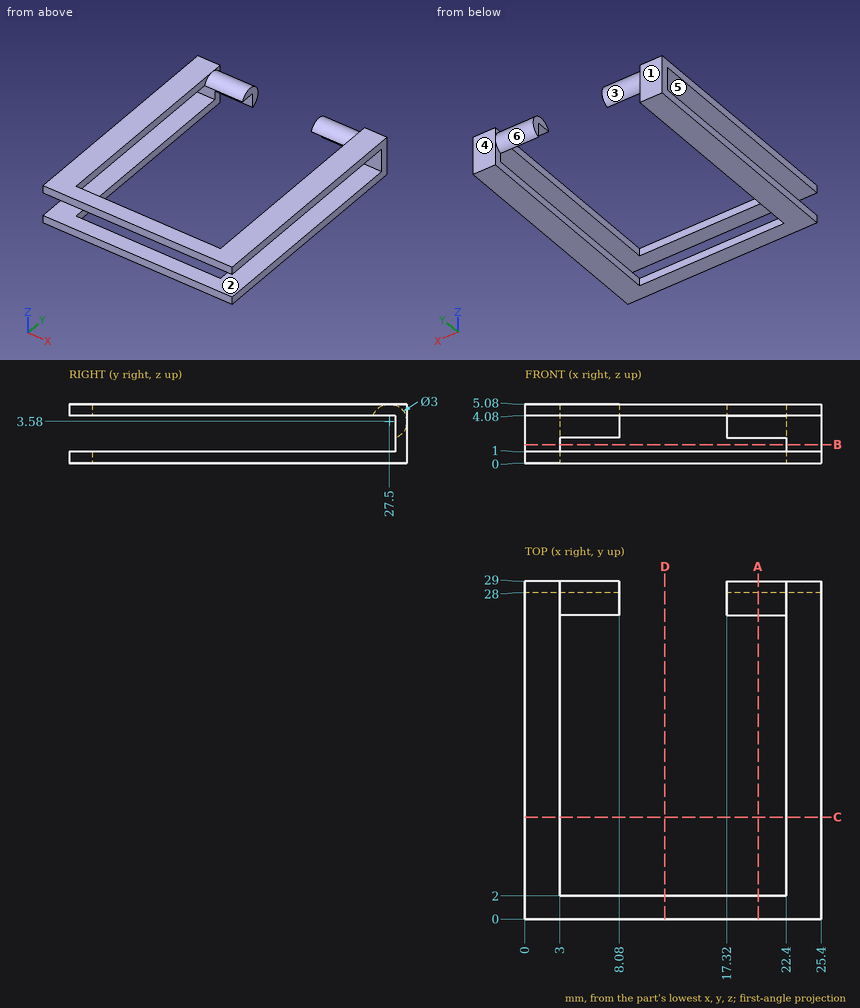
Answer from the drawing. Dimensions are ordinates in mm from the lowest x, y and z of the part. A direction names the side the tool comes from. Give positions to 0.01 mm unless a question says otherwise; leave off trailing zeros. Loops run counter-clockwise (first coordinate to the right, second up) from the corner with the lowest first, then second, coordinate; pieces in that order, holes last. Notation, with made-up numbers: (53, 64) - (59, 64) arc R20 cw to (59, 83) - close; hole circle Ø11 at (89, -31). An arc over 180 degrees is marked (long way). Write each question's results on one line, items separated by ' | '.
1. Find section B-B, the plane z = 1.6. Write down the section's boundary in (x, y), then the cut area to 3 significant figures.
Resolved:
outline: (0, 28) - (3, 28) - (3, 29) - (0, 29) - close; (22.4, 28) - (25.4, 28) - (25.4, 29) - (22.4, 29) - close | area: 6.00 mm^2
2. Which of the six approach directions +Z, -Z, +X, -X, +Y, -Y give full straight-line access (tool end or side, diameter ignored) to the marked faces 4, 5 and 6?
Resolved:
face 4: +Z, -Z, +X, -X, +Y | face 5: +X, -X, -Y | face 6: none
3. For a pull along Y with two mould halves and no side action, classify the marked faces 1, 2 and 3 as +Y half, -Y half, draft (parallel to the pull), parting line (faces both ways), or undercut.
Resolved:
face 1: +Y half | face 2: draft | face 3: undercut
4. Flat-ended cylindrical pins translate along their axes: P1, Ø1.5, axis at x = 22, z = 2, coming from the -Y side; P2, Ø0.5, axis at x = 13.5, z = 0.5, coming from the +Y side; P3, Ø0.9, axis at y = 27.5, z = 4, coming from the -X side. Find the tip coordinate at first contact, or state that the pin passes through.
Resolved:
P1: stops at y = 28 | P2: stops at y = 2 | P3: stops at x = 0
5. Find section C-C, the plane y = 8.75. Write down the section's boundary in (x, z), then the cut area to 3 significant figures.
Resolved:
outline: (0, 0) - (3, 0) - (3, 1) - (0, 1) - close; (0, 4.08) - (3, 4.08) - (3, 5.08) - (0, 5.08) - close; (22.4, 0) - (25.4, 0) - (25.4, 1) - (22.4, 1) - close; (22.4, 4.08) - (25.4, 4.08) - (25.4, 5.08) - (22.4, 5.08) - close | area: 12.0 mm^2
6. Consider probe 1 along Z at (x, y) = (2, 18.75); probe 2 along X at (y, z) = (23.5, 4.25); probe 3 along Y at (x, z) = (15, 4.55). Determine where each line is inside the solid, lowest interval first. Write a range as from..to.
Resolved:
probe 1: z = 0..1, 4.08..5.08 | probe 2: x = 0..3, 22.4..25.4 | probe 3: y = 0..2
7. Find section D-D, the plane x = 12. Write down the section's boundary in (y, z).
Resolved:
outline: (0, 0) - (2, 0) - (2, 1) - (0, 1) - close; (0, 4.08) - (2, 4.08) - (2, 5.08) - (0, 5.08) - close
8. Find section A-A, the plane x = 20. Write down the section's boundary in (y, z).
Resolved:
outline: (0, 0) - (2, 0) - (2, 1) - (0, 1) - close; (0, 4.08) - (2, 4.08) - (2, 5.08) - (0, 5.08) - close; (26.09, 4.08) - (28, 4.08) - (28, 2.17) arc R1.5 ccw (long way) to start
